```python
from build123d import *

# Parameters (mm, degrees)
F0_W     = 17.2
F0_H     = 8
F1_DEPTH = 8.1
F2_R     = 1.75
F3_DEPTH = 8.001
F4_R     = 2


with BuildPart() as f1:
    # F0 (on Front) → F1 (new body)
    with BuildSketch(Plane.XZ):
        with Locations((0, 4)):
            Rectangle(F0_W, F0_H)
    extrude(amount=F1_DEPTH)

    # F2 (on face) → F3 (cut, through all)
    with BuildSketch(Plane.XY.offset(8)):
        with Locations((-5.575, -4.05)):
            Circle(F2_R)
        with Locations((5.575, -4.05)):
            Circle(F2_R)
    extrude(amount=-F3_DEPTH, mode=Mode.SUBTRACT)

    # F4
    f4_edges = [f1.edges().sort_by_distance(p)[0] for p in [
        (-8.6, -8.1, 4),
        (8.6, -8.1, 4),
        (8.6, 0, 4),
        (-8.6, 0, 4),
    ]]
    fillet(f4_edges, radius=F4_R)


solid = f1.part
```
Verification items for the finished model (mm, model axes). Give positions to 0.01 mm unless a question says otherwise; leave off trailing zeros. Order: outer loops, then holes, each group sorted by start corner. A loop starts at its lowest first (then second) coordinate and runs counter-clockwise, first axis right, second up. Notation, with made-up numbers: M 28,26.25 L 40,26.25 A25 ccw 40,51.25 Z; hole C 75.5,39.25 d11. An arc over 180 degrees is marked long. Answer in a Markdown table with one row per item. Add a question column.
Item 1: Gauge pin test, flat ends, axial feed: pin 1 (2 mm diameter, centred on x = -5.575, y = -4.05, fed in from -Z); pin 2 (3 mm diameter, centred on x = 3.5, y = -4.5, fed in from -Z). Record the tip position at first contact, or that the pin passes through.
Item 2: Section check A-A, the plane y = -4.05. Enter the section's corners in (x, z) (3 decimals).
Item 3: Mould release check, pull along Y, two halves, no side actions. Record for faces 1 (the cylindrical face through (7.2, -4.7, 4.1)), 2 (the flat face through (0, -8.1, 4)), 3 (the flat face through (-8.6, -4, 4)), 4 (the cylindrical face through (8, -0.57, 4.06)): released by +Y, released by -Y, zero draft, split by the parting line, or undercut.
Item 4: Section check C-C, the plane x = 4. Enter the section's corners in (y, z), and give its area (3 significant figures).
Item 5: Section check D-D, the plane y = -7.5. Enter the section's corners in (x, z).
Item 6: Scan lines: probe 1 along X at (y, z) = (-2.5, 2.5); probe 2 along X at (y, z) = (-5.5, 1.25); probe 3 along Y at (x, z) = (6.75, 5). Record each from-to range of solid material in increasing order. Write a range as from..to.
Item 7: Section check B-B, the plane z = 7. Enter the section's corners in (x, y) (3 decimals).
Filled sheet:
| question | item | result |
|---|---|---|
| 1 | pin 1 | passes through |
| 1 | pin 2 | stops at z = 0 |
| 2 | outline | M -8.6,0 L -7.325,0 L -7.325,8 L -8.6,8 Z; M -3.825,0 L 3.825,0 L 3.825,8 L -3.825,8 Z; M 7.325,0 L 8.6,0 L 8.6,8 L 7.325,8 Z |
| 3 | face 1 | undercut |
| 3 | face 2 | released by -Y |
| 3 | face 3 | zero draft |
| 3 | face 4 | released by +Y |
| 4 | outline | M -8.1,0 L -4.81,0 L -4.81,8 L -8.1,8 Z; M -3.29,0 L 0,0 L 0,8 L -3.29,8 Z |
| 4 | area | 52.6 mm^2 |
| 5 | outline | M -8.03,0 L 8.03,0 L 8.03,8 L -8.03,8 Z |
| 6 | probe 1 | x = -8.6..-6.39, -4.76..4.76, 6.39..8.6 |
| 6 | probe 2 | x = -8.6..-6.55, -4.6..4.6, 6.55..8.6 |
| 6 | probe 3 | y = -8.09..-5.35, -2.75..-0.01 |
| 7 | outline | M -8.6,-6.1 A2 ccw -6.6,-8.1 L 6.6,-8.1 A2 ccw 8.6,-6.1 L 8.6,-2 A2 ccw 6.6,0 L -6.6,0 A2 ccw -8.6,-2 Z; hole C -5.575,-4.05 d3.5; hole C 5.575,-4.05 d3.5 |
